```python
from build123d import *
from build123d.topology import SkipClean

# Parameters (mm, degrees)
SKETCH2_R           = 3.475
BOSS_EXTRUDE2_DEPTH = 30.6846
SKETCH3_R           = 1.475
CUT_EXTRUDE1_DEPTH  = 10
CUT_EXTRUDE2_START  = -10
SKETCH4_R           = 1.475
CUT_EXTRUDE2_DEPTH  = 10
BOSS_EXTRUDE3_DEPTH = 30.6846
SKETCH6_W           = 6.95
SKETCH6_H           = 30.6846
BOSS_EXTRUDE4_DEPTH = 0.2
SKETCH8_W           = 3
SKETCH8_H           = 2
CUT_EXTRUDE3_DEPTH  = 32.675744698
SKETCH10_R          = 2.85
CUT_EXTRUDE4_DEPTH  = 3
SKETCH11_R          = 1.675
CUT_EXTRUDE5_DEPTH  = 32.138726849
BOSS_EXTRUDE5_REACH = 33.487
SKETCH12_R          = 4.85
SKETCH12_R_2        = 2.85
BOSS_EXTRUDE7_START = 1
SKETCH13_R          = 2.85
BOSS_EXTRUDE7_DEPTH = 1
CUT_EXTRUDE6_DEPTH  = 32.282148424
CUT_EXTRUDE7_DEPTH  = 32.877730235


with BuildPart() as part:
    # Sketch2 → Boss-Extrude2 (new body)
    with BuildSketch(Plane.XY):
        Circle(SKETCH2_R)
    extrude(amount=BOSS_EXTRUDE2_DEPTH)

    # Sketch3 → Cut-Extrude1 (cut)
    with BuildSketch(Plane.XY.offset(30.6846)):
        Circle(SKETCH3_R)
    extrude(amount=-CUT_EXTRUDE1_DEPTH, mode=Mode.SUBTRACT)

    # Sketch4 → Cut-Extrude2 (cut)
    with BuildSketch(Plane(origin=(0, 0, 0), x_dir=(-1, 0, 0), z_dir=(0, 0, -1)).offset(CUT_EXTRUDE2_START)):
        with Locations(Location((0, 0, 0), (0, 0, 180))):
            Circle(SKETCH4_R)
    extrude(amount=CUT_EXTRUDE2_DEPTH, mode=Mode.SUBTRACT)

    # Sketch5 → Boss-Extrude3 (add)
    with BuildSketch(Plane(origin=(0, 0, 0), x_dir=(-1, 0, 0), z_dir=(0, 0, -1))):
        with BuildLine():
            ThreePointArc((0, -3.475), (-2.457196065, -2.457196065), (-3.475, 0))
            Line((-3.475, 0), (-3.475, -3.475))
            Line((-3.475, -3.475), (0, -3.475))
        make_face()
        with BuildLine():
            Line((3.475, -3.475), (3.475, 0))
            ThreePointArc((3.475, 0), (2.457196065, -2.457196065), (0, -3.475))
            Line((0, -3.475), (3.475, -3.475))
        make_face()
    extrude(amount=-BOSS_EXTRUDE3_DEPTH)

    # Sketch6 → Boss-Extrude4 (add)
    with BuildSketch(Plane.XZ.offset(3.475)):
        with Locations((0, 15.3423)):
            Rectangle(SKETCH6_W, SKETCH6_H)
    extrude(amount=BOSS_EXTRUDE4_DEPTH)

    # Sketch8 → Cut-Extrude3 (cut, through all)
    with BuildSketch(Plane.ZY.offset(3.475)):
        with Locations((16.8423, 3.475)):
            Rectangle(SKETCH8_W, SKETCH8_H)
        with Locations((13.8423, 3.475)):
            Rectangle(SKETCH8_W, SKETCH8_H)
    extrude(amount=-CUT_EXTRUDE3_DEPTH, mode=Mode.SUBTRACT)

    # Sketch10 → Cut-Extrude4 (cut)
    with BuildSketch(Plane(origin=(0, 2.475, 0), x_dir=(1, 0, 0), z_dir=(0, 1, 0))):
        with Locations(Location((0, -15.3423, 0), (0, 0, 270))):
            Circle(SKETCH10_R)
    extrude(amount=-CUT_EXTRUDE4_DEPTH, mode=Mode.SUBTRACT)

    # Sketch11 → Cut-Extrude5 (cut, through all)
    with BuildSketch(Plane(origin=(0, -0.525, 0), x_dir=(1, 0, 0), z_dir=(0, 1, 0))):
        with Locations(Location((0, -15.3423, 0), (0, 0, 270))):
            Circle(SKETCH11_R)
    extrude(amount=-CUT_EXTRUDE5_DEPTH, mode=Mode.SUBTRACT)

    # Boss-Extrude5: up to this face of the body (flat: up to its plane)
    boss_extrude5_end = Plane(part.part.faces().sort_by_distance((0, -3.675, 30.369981632))[0])
    # Sketch12 → Boss-Extrude5 (add, up to the picked face)
    with BuildSketch(Plane(origin=(0, 2.475, 0), x_dir=(1, 0, 0), z_dir=(0, 1, 0)), mode=Mode.PRIVATE) as boss_extrude5_sk1:
        with Locations((0, -15.3423)):
            Circle(SKETCH12_R)
        with Locations(Location((0, -15.3423, 0), (0, 0, 270))):
            Circle(SKETCH12_R_2, mode=Mode.SUBTRACT)
    boss_extrude5_tool1 = split(extrude(boss_extrude5_sk1.sketch, amount=-BOSS_EXTRUDE5_REACH, mode=Mode.PRIVATE), bisect_by=boss_extrude5_end, keep=Keep.BOTH, mode=Mode.PRIVATE)
    add(boss_extrude5_tool1.solids().sort_by(Axis((-4.712821, 2.475, 15.3423), (0, -1, 0)))[0])

    # Sketch13 → Boss-Extrude7 (add)
    with BuildSketch(Plane(origin=(0, 2.475, 0), x_dir=(1, 0, 0), z_dir=(0, 1, 0)).offset(BOSS_EXTRUDE7_START)):
        with BuildLine():
            Line((-2.439262184, -19.534256584), (-2.439262184, -18.3423))
            Line((-2.439262184, -18.3423), (2.439262184, -18.3423))
            Line((2.439262184, -18.3423), (2.439262184, -19.534256584))
            ThreePointArc((2.439262184, -19.534256584), (4.85, -15.3423), (2.439262184, -11.150343416))
            Line((2.439262184, -11.150343416), (2.439262184, -12.3423))
            Line((2.439262184, -12.3423), (-2.439262184, -12.3423))
            Line((-2.439262184, -12.3423), (-2.439262184, -11.150343416))
            ThreePointArc((-2.439262184, -11.150343416), (-4.85, -15.3423), (-2.439262184, -19.534256584))
        make_face()
        with Locations(Location((0, -15.3423, 0), (0, 0, 270))):
            Circle(SKETCH13_R, mode=Mode.SUBTRACT)
    extrude(amount=-BOSS_EXTRUDE7_DEPTH)

    # Sketch15 → Cut-Extrude6 (cut, through all)
    with SkipClean():  # the faces are left unmerged after this step: merging them gives an invalid solid
        with BuildSketch(Plane(origin=(0, 0, 0), x_dir=(-1, 0, 0), z_dir=(0, 0, -1))):
            with BuildLine():
                Line((6.975728947, 0), (3.475, 0))
                ThreePointArc((3.475, 0), (0, 3.475), (-3.475, 0))
                Line((-3.475, 0), (-8.171324348, 0))
                Line((-8.171324348, 0), (-8.171324348, 6.073396115))
                Line((-8.171324348, 6.073396115), (6.975728947, 6.073396115))
                Line((6.975728947, 6.073396115), (6.975728947, 0))
            make_face()
        extrude(amount=-CUT_EXTRUDE6_DEPTH, mode=Mode.SUBTRACT)
    add(part.part.scale(1), mode=Mode.REPLACE)  # the faces are merged on a copy

    # Sketch16 → Cut-Extrude7 (cut, through all)
    with BuildSketch(Plane(origin=(0, -3.675, 0), x_dir=(-1, 0, 0), z_dir=(0, -1, 0))):
        Polygon((-3.475, -18.725623071), (-3.475, -11.958976929), (-9.441171238, -13.498522389), (-7.451050634, -19.072360919), align=None)
        Polygon((3.475, -18.725623071), (3.475, -11.958976929), (8.590567713, -11.958976929), (7.591441213, -18.725623071), align=None)
    extrude(amount=-CUT_EXTRUDE7_DEPTH, mode=Mode.SUBTRACT)


solid = part.part
```
Input: part model. Units: mm. Frame: model coordinates. A direction names the side the tool comes from. Give positions to 0.01 mm unless a question says otherwise; leave off trailing zeros. Order: outer loops, then holes, each group sorted by start corner. A loop starts at its lowest first (then second) coordinate and runs counter-clockwise, first axis right, second up. Notation, with made-up numbers: M 80.5,12 L 129.5,12 A34 cw 129.5,48 Z; hole C -20.5,41.25 d8. An arc over 180 degrees is marked long. One line per question, with ' | ' between items.
1) Section C-C on y = -1. Output: boundary loops of the cut face in (x, z) (3 decimals), and give its area (3 significant figures).
Filled in:
outline: M -3.475,0 L -1.084,0 L -1.084,10 L 1.084,10 L 1.084,0 L 3.475,0 L 3.475,30.685 L 1.084,30.685 L 1.084,20.685 L -1.084,20.685 L -1.084,30.685 L -3.475,30.685 Z; hole C 0,15.342 d3.35 | area: 161 mm2
2) Contact query for flat-ended pins moving along their axis: P1, Ø4, axis at x = 1.5, y = -1.5, coming from the -Z side; P2, Ø1.7, axis at x = 0, z = 14, coming from the +Y side (3 decimals); P3, Ø0.9, axis at x = 0.5, y = -0.5, coming from the +Z side; P4, Ø2.5, axis at x = 0, y = 0, coming from the -Z side. Output: stop coordinate, or through.
Filled in:
P1: stops at z = 0 | P2: stops at y = -0.525 | P3: stops at z = 20.68 | P4: stops at z = 10
3) Access query for faces 1 (the face through (-1, -0.525, 17)), 2 (the face through (0, 0, 20.685)), 3 (the face through (-1.474, -0.065, 5.07)). Directions: +Z, -Z, +X, -X, +Y, -Y. A direction counts if a zero-diameter tool reaches every point of the face in a straight line with its end or side. Return the directions, or none.
Filled in:
face 1: +Y | face 2: +Z | face 3: -Z
4) Section D-D on z = 3. Output: boundary loops of the cut face in (x, y) (3 decimals).
Filled in:
outline: M -3.475,-3.675 L 3.475,-3.675 L 3.475,0 A3.475 ccw -3.475,0 Z; hole C 0,0 d2.95
5) Ray query, L1, parallel to Z at x = 0, y = 1; L2, parallel to Z at x = 0, y = 2.45; L3, parallel to Y at x = 0, z = 6.5 (3 decimals). Return the intervals inside material, ascending.
Filled in:
L1: z = 10 to 12.49, 18.19 to 20.68 | L2: z = 0 to 12.49, 18.19 to 30.68 | L3: y = -3.675 to -1.475, 1.475 to 3.475
6) Draft query along X for faces 4 (the face through (2, -3.675, 16)), 5 (the face through (3.047, 1.671, 15.128)), 6 (the face through (-1.474, 0.065, 25.755)). Return one class per face: pulls with the +X half, pulls with the -X half, needs draft (parallel to the pull), parting line crosses it, or undercut.
Filled in:
face 4: needs draft | face 5: parting line crosses it | face 6: undercut
7) Section A-A on x = 0. Output: boundary loops of the cut face in (y, z) (3 decimals).
Filled in:
outline: M -3.675,0 L -1.475,0 L -1.475,10 L 1.475,10 L 1.475,0 L 3.475,0 L 3.475,12.492 L -0.525,12.492 L -0.525,13.667 L -3.675,13.667 Z; M -3.675,17.017 L -0.525,17.017 L -0.525,18.192 L 3.475,18.192 L 3.475,30.685 L 1.475,30.685 L 1.475,20.685 L -1.475,20.685 L -1.475,30.685 L -3.675,30.685 Z
8) Section B-B on y = 2.75. Output: boundary loops of the cut face in (x, z).
Filled in:
outline: M -2.12,0 L 2.12,0 L 2.12,13.44 A2.85 cw -2.12,13.44 Z; M -2.12,17.24 A2.85 cw 2.12,17.24 L 2.12,30.68 L -2.12,30.68 Z
